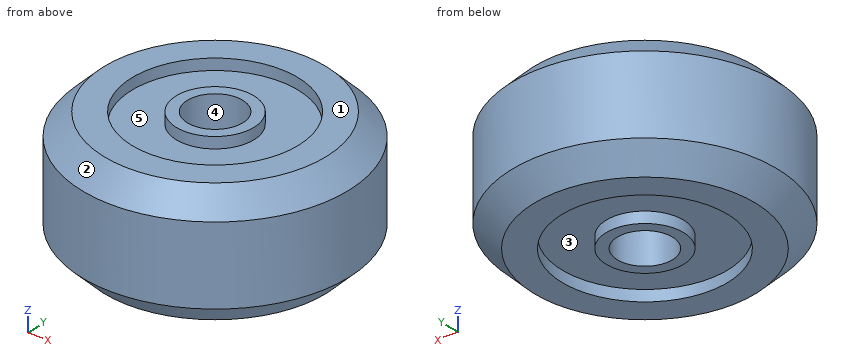
from build123d import *

# Parameters (mm, degrees)
SKETCH1_R           = 12
BOSS_EXTRUDE1_DEPTH = 11
CHAMFER1_SIZE       = 2
SKETCH2_R           = 2.5
CUT_EXTRUDE1_DEPTH  = 12
SKETCH3_R           = 7.5
SKETCH3_R_2         = 3.5
CUT_EXTRUDE2_DEPTH  = 1
SKETCH4_R           = 7.5
SKETCH4_R_2         = 3.5
CUT_EXTRUDE3_DEPTH  = 1


with BuildPart() as part:
    # Sketch1 → Boss-Extrude1 (new body)
    with BuildSketch(Plane.XY):
        Circle(SKETCH1_R)
    extrude(amount=BOSS_EXTRUDE1_DEPTH)

    # Chamfer1
    chamfer1_edges = [part.edges().sort_by_distance(p)[0] for p in [
        (-12, 0, 0),
        (-12, 0, 11),
    ]]
    chamfer(chamfer1_edges, length=CHAMFER1_SIZE)

    # Sketch2 → Cut-Extrude1 (cut, through all)
    with BuildSketch(Plane.XY.offset(11)):
        Circle(SKETCH2_R)
    extrude(amount=-CUT_EXTRUDE1_DEPTH, mode=Mode.SUBTRACT)

    # Sketch3 → Cut-Extrude2 (cut)
    with BuildSketch(Plane.XY.offset(11)):
        Circle(SKETCH3_R)
        Circle(SKETCH3_R_2, mode=Mode.SUBTRACT)
    extrude(amount=-CUT_EXTRUDE2_DEPTH, mode=Mode.SUBTRACT)

    # Sketch4 → Cut-Extrude3 (cut)
    with BuildSketch(Plane(origin=(0, 0, 0), x_dir=(-1, 0, 0), z_dir=(0, 0, -1))):
        Circle(SKETCH4_R)
        Circle(SKETCH4_R_2, mode=Mode.SUBTRACT)
    extrude(amount=-CUT_EXTRUDE3_DEPTH, mode=Mode.SUBTRACT)


solid = part.part
Input: part model. Units: mm. Frame: model coordinates. Face numbers are marked on the shaded views. A direction names the side the tool comes from. Round coordinates to 2 decimals unless told otherwise and drop trailing zeros. Write each loop counter-clockwise with the first axis right and the second up, starting at its lowest first coordinate (ties: lowest second). Pieces come first, ordered by that corner, then holes.
1) Cut plane A-A (y = 0). Return the cut outline in (x, z).
2) Draft query along X for the marked faces 1, 2 and 3. Return one class per face: pulls with the +X half, pulls with the -X half, needs draft (parallel to the pull), parting line crosses it, or undercut.
3) Ray query, L1, parallel to Y at x = 0, z = 2.5; L2, parallel to Y at x = 0, z = 0.7; L3, parallel to Z at x = 5.25, y = -1.5. Return the intervals inside material, ascending.
4) Cut plane D-D (z = 5.25). Return the cut outline in (x, y), then the cut area to 3 significant figures.
5) Cut plane C-C (z = 0.5). Return the cut outline in (x, y), then the cut area to 3 significant figures.
6) Reachability of the marked faces 4 and 5 from +Z, -Z, +X, -X, +Y, -Y: full face, straight path, thin tool, end or side. Return the list, or none.
7) Contact query for flat-ended pins moving along their axis: P1, Ø1.5, axis at y = 4.5, z = 2, coming from the -X side; P2, Ø1.5, axis at x = 5.5, y = -0.5, coming from the -Z side; P3, Ø6, axis at y = 5, z = 7.5, coming from the +X side. Output: stop coordinate, or through.
Geometry says:
1. outline: (-12, 2) - (-10, 0) - (-7.5, 0) - (-7.5, 1) - (-3.5, 1) - (-3.5, 0) - (-2.5, 0) - (-2.5, 11) - (-3.5, 11) - (-3.5, 10) - (-7.5, 10) - (-7.5, 11) - (-10, 11) - (-12, 9) - close; (2.5, 0) - (3.5, 0) - (3.5, 1) - (7.5, 1) - (7.5, 0) - (10, 0) - (12, 2) - (12, 9) - (10, 11) - (7.5, 11) - (7.5, 10) - (3.5, 10) - (3.5, 11) - (2.5, 11) - close
2. face 1: needs draft
2. face 2: parting line crosses it
2. face 3: undercut
3. L1: y = -12 to -2.5, 2.5 to 12
3. L2: y = -10.7 to -7.5, -3.5 to -2.5, 2.5 to 3.5, 7.5 to 10.7
3. L3: z = 1 to 10
4. outline: circle Ø24 at (0, 0); hole circle Ø5 at (0, 0)
4. area: 433 mm2
5. outline: circle Ø21 at (0, 0); circle Ø7 at (0, 0); hole circle Ø15 at (0, 0); hole circle Ø5 at (0, 0)
5. area: 188 mm2
6. face 4: +Z, -Z
6. face 5: +Z
7. P1: stops at x = -11.4
7. P2: stops at z = 1
7. P3: stops at x = 11.83
